Read the model definition and answer for the solid it produces. Units are mm, in the model's axes. Coordinates: 2 decimals unless noted, no trailing zeros. Write each loop counter-clockwise with the first axis right and the second up, starting at its lowest first coordinate (ties: lowest second). Pieces come first, ordered by that corner, then holes.
(1) The part is cut by section B-B, the plane x = 37.5. Determine the outline of the cut face in (y, z) (3 decimals).
(2) The part is cut by section C-C, the plane y = 2.4. State how many separate pieces and enclosed holes the cut face has, and give its area (3 significant figures).
(3) The part is cut by section D-D, the plane x = -47.5. Determine the outline of the cut face in (y, z) (3 decimals), and give its area (3 significant figures).
(4) Given pin 1 (4 mm diameter, centred on x = -50, z = 39, fed in from -Y); pin 2 (1 mm diameter, centred on y = 2, z = 41.5, fed in from -X); pin 3 (1.6 mm diameter, centred on y = 1.5, z = -3.5, fed in from +X), each flat-ended and moving along its own axis, determine where each tip first touches the part or whether it passes through.
(5) Straight lines are drawn through the part: line 1 along Z through (x, y) = (5, 1.3); line 2 along Z through (x, y) = (-0.5, 2.7); line 3 along Z through (x, y) = (12, 0.75). For each, find the intervals that lie inside material, in ascending order.
(6) The part is cut by section A-A, the plane z = 57.15. Determine the outline of the cut face in (x, y) (3 decimals), and give its area (3 significant figures).
(7) Determine the mould class of faces 1 (the flat face through (0, 2, 68.072)), 2 (the flat face through (-68.072, 2, 0)), 3 (the flat face through (-15, 0, -1)) for opening direction X: pulls with the +X half, pulls with the -X half, needs draft (parallel to the pull), parting line crosses it, or undercut.
```python
from build123d import *

# Parameters (mm, degrees)
SKETCH1_R                       = 74.422
SKETCH1_W                       = 21.200000018
SKETCH1_H                       = 41.29999995
BOSS_EXTRUDE1_DEPTH             = 3.175
F_4_6_4_6_DIAMETER_HOLE1_D      = 4.6
F_4_CLEARANCE_HOLE1_D           = 3.2639
CIRPATTERN2_COUNT               = 4
F_1_4_CLEARANCE_HOLE1_D         = 7.14248
SKETCH19_W                      = 19.05
SKETCH19_H                      = 12.7
CUT_EXTRUDE1_DEPTH              = 106.29648044
CIRPATTERN3_COUNT               = 4
FILLET1_R                       = 1.27
F_19_0_166_DIAMETER_HOLE1_D     = 4.2164
TAP_DRILL_FOR_M3X0_5_TAP1_D     = 2.5
TAP_DRILL_FOR_M3X0_5_TAP1_DEPTH = 3.81
TAP_DRILL_FOR_M3X0_5_TAP1_TIP   = 0.751075774


with BuildPart() as part:
    # Sketch1 → Boss-Extrude1 (new body)
    with BuildSketch(Plane(origin=(0, 0, 0), x_dir=(1, 0, 0), z_dir=(0, 1, 0))):
        with Locations(Location((0, 0, 0), (0, 0, 270))):
            Circle(SKETCH1_R)
        with Locations((0, -10.649999909)):
            Rectangle(SKETCH1_W, SKETCH1_H, mode=Mode.SUBTRACT)
    extrude(amount=BOSS_EXTRUDE1_DEPTH)

    # Ø4.6 (4.6) Diameter Hole1 (through all)
    with Locations(Plane(origin=(0, 0, 0), x_dir=(-1, 0, 0), z_dir=(0, -1, 0))):
        with Locations((-5.000000033, 13.350000097), (4.999999906, 13.350000097), (-5.000000033, -34.649999915), (4.999999906, -34.649999915)):
            Hole(F_4_6_4_6_DIAMETER_HOLE1_D / 2)

    # #4 Clearance Hole1 (through all)
    with Locations(Plane(origin=(0, 0, 0), x_dir=(-1, 0, 0), z_dir=(0, -1, 0))):
        with Locations((60.506475165, -29.075578741), (29.075578741, -60.506475165), (11.115066499, -42.545962923), (20.09532262, -51.526219044), (51.526219044, -20.09532262), (42.545962923, -11.115066499)):
            f_4_clearance_hole1 = Hole(F_4_CLEARANCE_HOLE1_D / 2)

    # CirPattern2: #4 Clearance Hole1 ×4 about axis
    cirpattern2_axis = Axis((0, 0, 0), (0, 1, 0))
    for i in range(1, CIRPATTERN2_COUNT):
        add(f_4_clearance_hole1.rotate(cirpattern2_axis, i * 360 / CIRPATTERN2_COUNT), mode=Mode.SUBTRACT)

    # 1/4 Clearance Hole1 (through all)
    with Locations(Plane(origin=(0, 3.175, 0), x_dir=(1, 0, 0), z_dir=(0, 1, 0))):
        with Locations((0, 57.15), (0, -57.15)):
            Hole(F_1_4_CLEARANCE_HOLE1_D / 2)

    # Sketch19 → Cut-Extrude1 (cut, through all)
    with BuildSketch(Plane.XZ):
        with Locations((0, -74.422)):
            Rectangle(SKETCH19_W, SKETCH19_H)
    cut_extrude1 = extrude(amount=-CUT_EXTRUDE1_DEPTH, mode=Mode.SUBTRACT)

    # CirPattern3: Cut-Extrude1 ×4 about axis
    cirpattern3_axis = Axis((0, 0, 0), (0, 1, 0))
    for i in range(1, CIRPATTERN3_COUNT):
        add(cut_extrude1.rotate(cirpattern3_axis, i * 360 / CIRPATTERN3_COUNT), mode=Mode.SUBTRACT)

    # Fillet1
    fillet1_edges = [part.edges().sort_by_distance(p)[0] for p in [
        (-9.525, 1.5875, -73.809948239),
        (9.525, 1.5875, -73.809948239),
        (9.525, 1.5875, -68.072),
        (-9.525, 1.5875, -68.072),
        (73.809948239, 1.5875, -9.525),
        (73.809948239, 1.5875, 9.525),
        (9.525, 1.5875, 73.809948239),
        (-9.525, 1.5875, 73.809948239),
        (-73.809948239, 1.5875, 9.525),
        (-73.809948239, 1.5875, -9.525),
        (-68.072, 1.5875, -9.525),
        (-68.072, 1.5875, 9.525),
        (-9.525, 1.5875, 68.072),
        (9.525, 1.5875, 68.072),
        (68.072, 1.5875, 9.525),
        (68.072, 1.5875, -9.525),
        (10.600000009, 1.5875, 31.299999884),
        (10.600000009, 1.5875, -10.000000066),
        (-10.600000009, 1.5875, -10.000000066),
        (-10.600000009, 1.5875, 31.299999884),
    ]]
    fillet(fillet1_edges, radius=FILLET1_R)

    # #19 (0.166) Diameter Hole1 (through all)
    with Locations(Plane(origin=(0, 3.175, 0), x_dir=(1, 0, 0), z_dir=(0, 1, 0))):
        with Locations((-16.963217712, 68.448703271), (-64.109562348, 15.914204963), (-57.823383063, 9.628025678)):
            Hole(F_19_0_166_DIAMETER_HOLE1_D / 2)

    # Tap Drill for M3x0.5 Tap1
    with Locations(Plane(origin=(0, 3.175, 0), x_dir=(1, 0, 0), z_dir=(0, 1, 0))):
        with Locations((18.220000103, 5.225000097), (18.220000103, -20.174999903), (32.190000103, -1.124999903)):
            Hole(TAP_DRILL_FOR_M3X0_5_TAP1_D / 2, depth=TAP_DRILL_FOR_M3X0_5_TAP1_DEPTH)
            with Locations((0, 0, -(TAP_DRILL_FOR_M3X0_5_TAP1_DEPTH + TAP_DRILL_FOR_M3X0_5_TAP1_TIP / 2))):  # 118° drill point
                Cone(0, TAP_DRILL_FOR_M3X0_5_TAP1_D / 2, TAP_DRILL_FOR_M3X0_5_TAP1_TIP, mode=Mode.SUBTRACT)


solid = part.part
```
Computed:
1. outline: (0, -64.284) - (3.175, -64.284) - (3.175, 64.284) - (0, 64.284) - close
2. separate pieces: 1
2. enclosed holes: 37
2. area: 15,700 mm2
3. outline: (0, -57.292) - (3.175, -57.292) - (3.175, 57.292) - (0, 57.292) - close
3. area: 364 mm2
4. pin 1: stops at y = 0
4. pin 2: stops at x = -62.11
4. pin 3: stops at x = 68.07
5. line 1: z = -68.07 to -15.65, -11.05 to -10, 31.3 to 32.35, 36.95 to 68.07
5. line 2: z = -68.07 to -60.69, -53.61 to -10, 31.3 to 53.61, 60.69 to 68.07
5. line 3: z = -73.45 to -43.92, -41.17 to 41.17, 43.92 to 73.45
6. outline: (-47.671, 0) - (-3.571, 0) - (-3.571, 3.175) - (-47.671, 3.175) - close; (3.571, 0) - (47.671, 0) - (47.671, 3.175) - (3.571, 3.175) - close
6. area: 280 mm2
7. face 1: undercut
7. face 2: pulls with the -X half
7. face 3: needs draft
